Could you check a few things on this drawing? It's one solid part, dimensions in mm from its lowest x, y, z. A direction names the side the tool comes from. Give positions to 0.01 mm unless a question says otherwise; leave off trailing zeros. Loops run counter-clockwise (first coordinate to the right, second up) from the corner with the lowest first, then second, coordinate; pieces in that order, holes last. Notation, with made-up numbers: (52, 56.5) -> (58, 56.5) arc R36 cw to (58, 94.5) -> close; hole circle Ø3 at (67.5, 35.5). An arc over 180 degrees is marked (long way). Use CSV: the item, a comma, the result in double quotes.
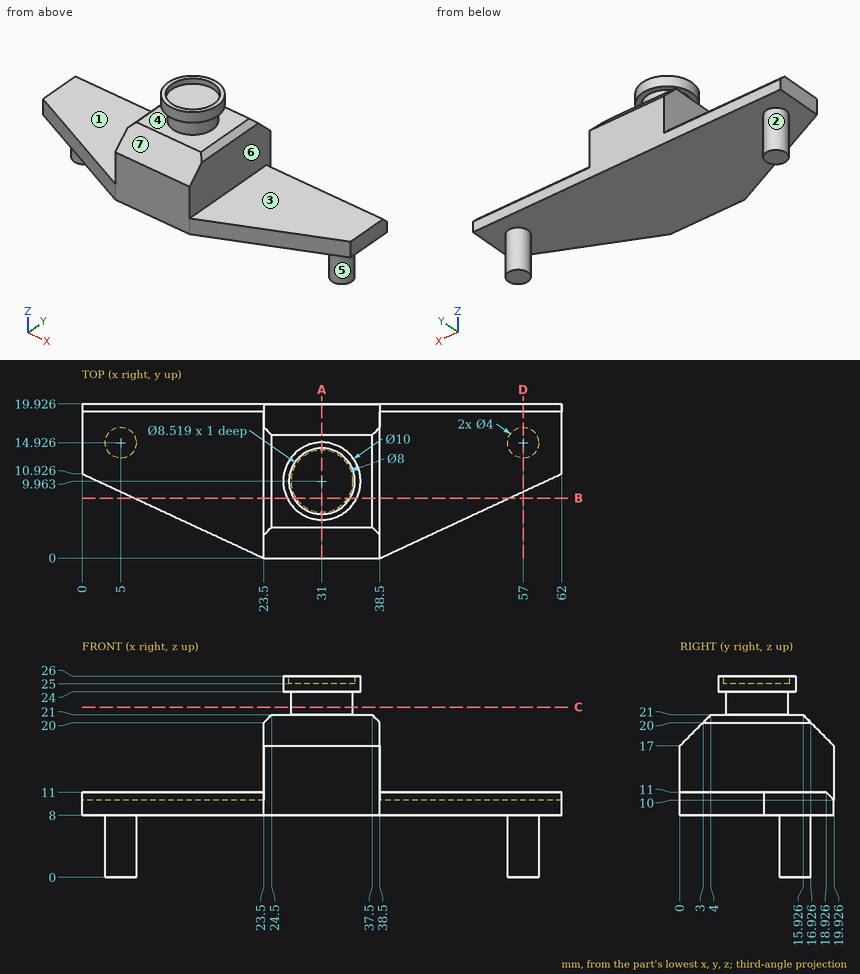
(1) If we section it at D-D, the plane x = 57: Write out the boundary of the cut face in (y, z) (1 decimal).
Answer sheet:
outline,"(8.6, 8) -> (12.9, 8) -> (12.9, 0) -> (16.9, 0) -> (16.9, 8) -> (19.9, 8) -> (19.9, 10) -> (18.9, 11) -> (8.6, 11) -> close"
(2) Which directions (+Z, -Z, +X, -X, +Y, -Y) give clear straight access to the entire face, cutting with the end or side of a thin tool? Please do the marked faces 1, 2, 3 and 4.
Answer sheet:
face 1,"+Z, -X, +Y, -Y"
face 2,"-Z"
face 3,"+Z, +X, +Y, -Y"
face 4,"none"
(3) We'd pull the mould along X, two halves only. Please class the marked faces 5, 6 and 7: released by +X, released by -X, zero draft, split by the parting line, or undercut.
Answer sheet:
face 5,"undercut"
face 6,"released by +X"
face 7,"zero draft"
(4) If we section it at C-C, the plane z = 22: Write out the boundary of the cut face in (x, y).
Answer sheet:
outline,"circle Ø8 at (31, 9.96)"
(5) If I drill on L1, parallel to Y at x = 31, z = 25.75; L2, parallel to Z at x = 15, y = 10; L3, parallel to Z at x = 34, y = 12, over which ranges is the centre line in solid material (lowest first)? Write a range as from..to.
Answer sheet:
L1,"y = 4.96..5.7, 14.22..14.96"
L2,"z = 8..11"
L3,"z = 8..25"
(6) Will these pins go through, and if not, where does the flat tip stop? pin 1 Ø9.5 at (x, y) = (10, 11.5) entering from +Z; pin 2 Ø8 at (y, z) = (14.5, 16) entering from -X; pin 3 Ø3 at (x, y) = (31.5, 11.5) entering from -Z.
Answer sheet:
pin 1,"stops at z = 11"
pin 2,"stops at x = 23.5"
pin 3,"stops at z = 8"
(7) If we section it at B-B, the plane y = 7.75: Write out the boundary of the cut face in (x, z).
Answer sheet:
outline,"(6.83, 8) -> (55.17, 8) -> (55.17, 11) -> (38.5, 11) -> (38.5, 20) -> (37.5, 21) -> (34.33, 21) -> (34.33, 24) -> (35.48, 24) -> (35.48, 26) -> (34.64, 26) -> (34.64, 25) -> (27.36, 25) -> (27.36, 26) -> (26.52, 26) -> (26.52, 24) -> (27.67, 24) -> (27.67, 21) -> (24.5, 21) -> (23.5, 20) -> (23.5, 11) -> (6.83, 11) -> close"
(8) If we section it at A-A, the plane x = 31: Write out the boundary of the cut face in (y, z) (1 decimal).
Answer sheet:
outline,"(0, 8) -> (19.9, 8) -> (19.9, 17) -> (15.9, 21) -> (14, 21) -> (14, 24) -> (15, 24) -> (15, 26) -> (14.2, 26) -> (14.2, 25) -> (5.7, 25) -> (5.7, 26) -> (5, 26) -> (5, 24) -> (6, 24) -> (6, 21) -> (4, 21) -> (0, 17) -> close"
